from build123d import *

# Parameters (mm, degrees)
BOSS_EXTRUDE1_DEPTH   = 2.4
FILLET1_R             = 1
SKETCH3_R             = 1.9225
BOSS_EXTRUDE2_DEPTH   = 141
KES_EKSTR_ZYON1_DEPTH = 0.06


with BuildPart() as part:
    # Sketch1 → Boss-Extrude1 (new body)
    with BuildSketch(Plane(origin=(0, 0, 0), x_dir=(1, 0, 0), z_dir=(0, 1, 0))):
        with BuildLine():
            Line((-15, 3.25), (-9.45714016, 3.25))
            ThreePointArc((-9.45714016, 3.25), (-7.071067812, 7.071067812), (-3.25, 9.45714016))
            Line((-3.25, 9.45714016), (-3.25, 15))
            ThreePointArc((-3.25, 15), (0, 18.25), (3.25, 15))
            Line((3.25, 15), (3.25, 9.45714016))
            ThreePointArc((3.25, 9.45714016), (7.071067812, 7.071067812), (9.45714016, 3.25))
            Line((9.45714016, 3.25), (15, 3.25))
            ThreePointArc((15, 3.25), (18.25, 0), (15, -3.25))
            Line((15, -3.25), (9.45714016, -3.25))
            ThreePointArc((9.45714016, -3.25), (7.071067812, -7.071067812), (3.25, -9.45714016))
            Line((3.25, -9.45714016), (3.25, -15))
            ThreePointArc((3.25, -15), (0, -18.25), (-3.25, -15))
            Line((-3.25, -15), (-3.25, -9.45714016))
            ThreePointArc((-3.25, -9.45714016), (-7.071067812, -7.071067812), (-9.45714016, -3.25))
            Line((-9.45714016, -3.25), (-15, -3.25))
            ThreePointArc((-15, -3.25), (-18.25, 0), (-15, 3.25))
        make_face()
        with BuildLine():
            Line((-15, 1.42), (-9.5, 1.42))
            ThreePointArc((-9.5, 1.42), (-8.08, 0), (-9.5, -1.42))
            Line((-9.5, -1.42), (-15, -1.42))
            ThreePointArc((-15, -1.42), (-16.42, 0), (-15, 1.42))
        make_face(mode=Mode.SUBTRACT)
        with BuildLine():
            Line((1.42, 15), (1.42, 9.5))
            ThreePointArc((1.42, 9.5), (0, 8.08), (-1.42, 9.5))
            Line((-1.42, 9.5), (-1.42, 15))
            ThreePointArc((-1.42, 15), (0, 16.42), (1.42, 15))
        make_face(mode=Mode.SUBTRACT)
        with BuildLine():
            Line((15, -1.42), (9.5, -1.42))
            ThreePointArc((9.5, -1.42), (8.08, 0), (9.5, 1.42))
            Line((9.5, 1.42), (15, 1.42))
            ThreePointArc((15, 1.42), (16.42, 0), (15, -1.42))
        make_face(mode=Mode.SUBTRACT)
        with BuildLine():
            Line((-1.42, -15), (-1.42, -9.5))
            ThreePointArc((-1.42, -9.5), (0, -8.08), (1.42, -9.5))
            Line((1.42, -9.5), (1.42, -15))
            ThreePointArc((1.42, -15), (0, -16.42), (-1.42, -15))
        make_face(mode=Mode.SUBTRACT)
    extrude(amount=BOSS_EXTRUDE1_DEPTH)

    # Fillet1
    fillet1_edges = [part.edges().sort_by_distance(p)[0] for p in [
        (-9.45714016, 1.2, -3.25),
        (-3.25, 1.2, -9.45714016),
        (3.25, 1.2, -9.45714016),
        (9.45714016, 1.2, -3.25),
        (9.45714016, 1.2, 3.25),
        (3.25, 1.2, 9.45714016),
        (-3.25, 1.2, 9.45714016),
        (-9.45714016, 1.2, 3.25),
    ]]
    fillet(fillet1_edges, radius=FILLET1_R)

    # Sketch2 → Revolve1 (revolve)
    with BuildSketch(Plane.XY):
        with BuildLine():
            Line((1.925, 29.7), (2.464294328, 29.7))
            ThreePointArc((2.464294328, 29.7), (4.04285617, 29.138592921), (4.912445377, 27.70651401))
            Line((4.912445377, 27.70651401), (7.5, 15.2))
            Line((7.5, 15.2), (7.5, 2.4))
            Line((7.5, 2.4), (5.625, 2.4))
            Line((5.625, 2.4), (5.625, 15.2))
            Line((5.625, 15.2), (3.404891948, 26.194820827))
            ThreePointArc((3.404891948, 26.194820827), (2.889371485, 27.2829386), (1.925, 28.003874988))
            Line((1.925, 28.003874988), (1.925, 29.7))
        make_face()
    revolve(axis=Axis((0, 2.4, 0), (0, 1, 0)))

    # Sketch3 → Boss-Extrude2 (add)
    with BuildSketch(Plane(origin=(0, 2.4, 0), x_dir=(1, 0, 0), z_dir=(0, 1, 0))):
        Circle(SKETCH3_R)
    extrude(amount=BOSS_EXTRUDE2_DEPTH)

    # Sketch4 → Revolve2 (revolve)
    with BuildSketch(Plane(origin=(0, 0, 0), x_dir=(0, 0, -1), z_dir=(1, 0, 0))):
        with BuildLine():
            Line((6.922649731, 142.4), (3.230934575, 136.005761782))
            ThreePointArc((3.230934575, 136.005761782), (2.938114252, 135.712941459), (2.538114252, 135.605761782))
            Line((2.538114252, 135.605761782), (1.9225, 135.605761782))
            Line((1.9225, 135.605761782), (1.9225, 143.4))
            Line((1.9225, 143.4), (0, 143.4))
            Line((0, 143.4), (0, 144.9))
            Line((0, 144.9), (17.5, 144.9))
            Line((17.5, 144.9), (17.5, 143.4))
            Line((17.5, 143.4), (8.654700538, 143.4))
            ThreePointArc((8.654700538, 143.4), (7.654700538, 143.132050808), (6.922649731, 142.4))
        make_face()
    revolve(axis=Axis((0, 143.4, 0), (0, -1, 0)))

    # Çizim1 → Kes-Ekstrüzyon1 (cut)
    with BuildSketch(Plane.XZ.offset(-143.4)):
        Polygon((2.473531895, 11.056579199), (2.409957676, 10.172692481), (0.082320957, 10.339489356), (0.334567051, 13.859997168), (2.66220377, 13.693200293), (2.599313145, 12.809997168), (1.511715488, 12.887926856), (1.480270176, 12.451794043), (2.237008457, 12.397790137), (2.173434238, 11.513903418), (1.416695957, 11.567907324), (1.385934238, 11.134508887), align=None)
        Polygon((3.792276096, 9.57689352), (2.680752659, 10.121717739), (5.101358127, 12.856776332), (6.685244846, 12.080213832), (6.008487034, 8.490663051), (4.89764719, 9.034803676), (5.015225315, 9.640467739), (4.199014377, 10.040370082), align=None)
        Polygon((4.76639719, 10.68704977), (5.177920627, 10.485389614), (5.35702219, 11.371327114), align=None, mode=Mode.SUBTRACT)
        with BuildLine():
            Line((10.49023887, 8.045909213), (9.301469339, 7.814170932))
            add(Edge.make_bspline(
                [(9.301469339, 7.814170932), (9.295162601, 7.849093276), (9.282863589, 7.91719668), (9.259765757, 8.016165899), (9.231766875, 8.109044475), (9.199649304, 8.196046435), (9.163730366, 8.277260103), (9.122086055, 8.351638268), (9.078384744, 8.421598141), (9.044202502, 8.463454613), (9.027348245, 8.484092807)],
                knots=[0, 0, 0, 0, 0.000106452, 0.000207596, 0.000304698, 0.000397269, 0.000485696, 0.00057075, 0.000652855, 0.000732716, 0.000732716, 0.000732716, 0.000732716], degree=3))
            add(Edge.make_bspline(
                [(9.027348245, 8.484092807), (9.01594409, 8.496831925), (8.993668142, 8.52171548), (8.957180327, 8.554902215), (8.918891069, 8.58263641), (8.879448715, 8.606805989), (8.837738681, 8.624547904), (8.795060394, 8.639748228), (8.750352942, 8.648261409), (8.689312805, 8.653650441), (8.61134576, 8.649600922), (8.51970475, 8.622824869), (8.429383641, 8.578500593), (8.375376925, 8.535791651), (8.347172464, 8.513487338)],
                knots=[0, 0, 0, 0, 5.1274e-05, 0.000100155, 0.000147599, 0.000192969, 0.000238571, 0.000283319, 0.000328632, 0.000374616, 0.000467063, 0.000560776, 0.000659216, 0.00076682, 0.00076682, 0.00076682, 0.00076682], degree=3))
            add(Edge.make_bspline(
                [(8.347172464, 8.513487338), (8.32238698, 8.49082732), (8.275523945, 8.447982998), (8.221828166, 8.374475546), (8.186518469, 8.299074978), (8.171541706, 8.220584969), (8.176882746, 8.140146557), (8.201970979, 8.058369087), (8.24745169, 7.976028431), (8.288027536, 7.924336237), (8.309574808, 7.896885776)],
                knots=[0, 0, 0, 0, 0.000100546, 0.000190108, 0.000271179, 0.000348404, 0.000427163, 0.000510645, 0.000603011, 0.000707603, 0.000707603, 0.000707603, 0.000707603], degree=3))
            Line((8.309574808, 7.896885776), (8.728617776, 8.253038119))
            Line((8.728617776, 8.253038119), (9.527055276, 7.314463901))
            Line((9.527055276, 7.314463901), (8.085356058, 6.088096713))
            add(Edge.make_bspline(
                [(8.085356058, 6.088096713), (8.043412666, 6.130918963), (7.963019255, 6.212996893), (7.848036495, 6.330909372), (7.745125301, 6.439426088), (7.651824198, 6.535975119), (7.570495488, 6.623033205), (7.499975002, 6.699500807), (7.440576701, 6.765659164), (7.404913451, 6.806519435), (7.388774026, 6.825010776)],
                knots=[0, 0, 0, 0, 0.000179825, 0.000344674, 0.000494074, 0.000628484, 0.000747456, 0.000851473, 0.000940545, 0.001014176, 0.001014176, 0.001014176, 0.001014176], degree=3))
            add(Edge.make_bspline(
                [(7.388774026, 6.825010776), (7.362058603, 6.85691328), (7.309444418, 6.919743064), (7.236989178, 7.015916122), (7.169853497, 7.110629262), (7.110069184, 7.204873936), (7.055748887, 7.297651818), (7.008392801, 7.389665379), (6.967289467, 7.480685486), (6.932054654, 7.570889978), (6.904285219, 7.660554079), (6.881879716, 7.748984602), (6.867047818, 7.836567991), (6.8580281, 7.923104859), (6.855033423, 8.008796842), (6.859351934, 8.093567562), (6.869528685, 8.177437845), (6.89179563, 8.287308778), (6.930587621, 8.421570582), (6.989518301, 8.577515834), (7.059974362, 8.728287923), (7.144056677, 8.87248116), (7.238974286, 9.012055008), (7.347673596, 9.144627972), (7.468154157, 9.271895089), (7.556552427, 9.35016865), (7.601371683, 9.389854526)],
                knots=[0, 0, 0, 0, 0.000124813, 0.000245811, 0.00036112, 0.000473004, 0.00058052, 0.000683552, 0.000783294, 0.000880029, 0.000973863, 0.001064719, 0.001153502, 0.001240092, 0.001325585, 0.00141045, 0.001494477, 0.001578803, 0.001746506, 0.001913085, 0.002078523, 0.002245136, 0.00241332, 0.002584355, 0.002758907, 0.002938427, 0.002938427, 0.002938427, 0.002938427], degree=3))
            add(Edge.make_bspline(
                [(7.601371683, 9.389854526), (7.633267182, 9.416124727), (7.696616127, 9.468301038), (7.794804449, 9.540632275), (7.89522225, 9.606383047), (7.996644151, 9.666761034), (8.100532816, 9.720065252), (8.205586837, 9.768027651), (8.312583613, 9.809888085), (8.420955565, 9.84541849), (8.529824651, 9.873991879), (8.63797322, 9.895680951), (8.744963509, 9.908130177), (8.850675885, 9.915266481), (8.955311133, 9.911662891), (9.058901226, 9.902751782), (9.161192476, 9.884483788), (9.262208706, 9.859340021), (9.361575353, 9.826665303), (9.457961526, 9.785512166), (9.551318063, 9.73663609), (9.641991537, 9.680468107), (9.72947251, 9.615894492), (9.814300197, 9.543841789), (9.89671096, 9.464752006), (9.947642677, 9.406869871), (9.973441995, 9.377549838)],
                knots=[0, 0, 0, 0, 0.000123949, 0.000246181, 0.000365628, 0.000483921, 0.000600102, 0.000715741, 0.000830244, 0.0009446, 0.001057681, 0.001167748, 0.001275177, 0.00138063, 0.001485255, 0.001588921, 0.001692315, 0.001796601, 0.001901012, 0.002005762, 0.002110638, 0.002216866, 0.002325426, 0.002436499, 0.002550592, 0.002667712, 0.002667712, 0.002667712, 0.002667712], degree=3))
            add(Edge.make_bspline(
                [(9.973441995, 9.377549838), (10.008964061, 9.333535211), (10.080876677, 9.244429836), (10.173686342, 9.096785456), (10.258402353, 8.938194374), (10.331918381, 8.768701017), (10.393760496, 8.59235643), (10.441989787, 8.412398366), (10.475629511, 8.230183983), (10.485369339, 8.107330913), (10.49023887, 8.045909213)],
                knots=[0, 0, 0, 0, 0.000169553, 0.000343252, 0.000522153, 0.000708588, 0.000896894, 0.001082278, 0.001267051, 0.001451795, 0.001451795, 0.001451795, 0.001451795], degree=3))
        make_face()
    extrude(amount=-KES_EKSTR_ZYON1_DEPTH, mode=Mode.SUBTRACT)


solid = part.part
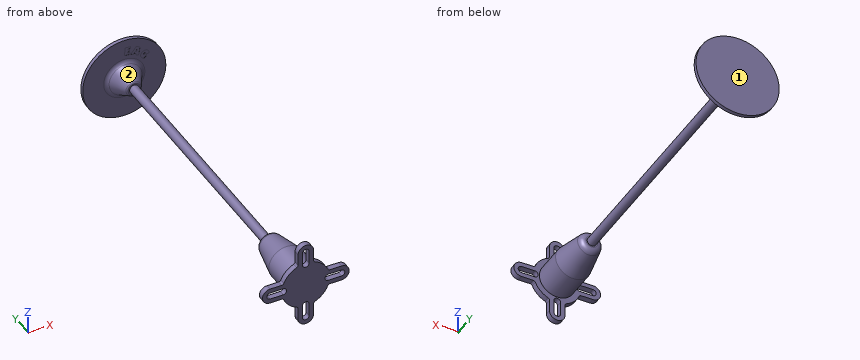
CAD build for the part. Positions are in the model's coordinates, mm. Face numbers are marked on the shaded views. A direction names the side the tool comes from. Round coordinates to 2 decimals unless told otherwise and drop trailing zeros. Order: outer loops, then holes, each group sorted by start corner. A loop starts at its lowest first (then second) coordinate and runs counter-clockwise, first axis right, second up. Notation, with made-up numbers: (2, -31.75) -> (29, -31.75) arc R23 ccw to (29, 7.25) -> close; hole circle Ø8 at (39, 67.5). An arc over 180 degrees is marked (long way). Write item = value, one per line. Start each with the question number.
(1) Cut at B-B, the plane x = -12.5. List the corners of the cut face in (y, z), then the cut area to 3 significant figures.
(2) Cut at D-D, the plane y = 51.5. List the corners of the cut face in (x, z) (1 decimal), then the cut area to 3 significant figures.
(3) Cut at A-A, the plane y = 11.5. State how many separate pieces and enclosed holes the cut face has, then the cut area to 3 significant figures.
(4) Which spindle directions (+Z, -Z, +X, -X, +Y, -Y) get a long thin tool onto all of the face, cutting with end or side? Do the marked faces 1 and 2. Say none if no direction does.
(5) Pin check, flat tips, straight feed: P1, Ø1.9, axis at y = 1, z = 12, coming from the +X side; P2, Ø2.5, axis at y = 1.5, z = -13, coming from the -X side; P3, Ø1.9, axis at x = 12.5, y = 1.5, coming from the +Z side. Stop position of each tip, or through.
(6) Probe line 1 (X direction, y = 8, z = 0) (1 decimal); line 2 (Y direction, x = 1.5, z = 1.5); line 3 (Y direction, x = -0.5, z = -16.5). List the from-to ranges inside material, lowest first. Write a range as [from, to].
Model answer:
q1.outline = (0, -3.25) -> (2.4, -3.25) -> (2.4, -1.42) -> (0, -1.42) -> close; (0, 1.42) -> (2.4, 1.42) -> (2.4, 3.25) -> (0, 3.25) -> close; (143.4, -12.25) -> (144.9, -12.25) -> (144.9, 12.25) -> (143.4, 12.25) -> close
q1.area = 45.5 mm2
q2.outline = circle Ø3.8 at (0, 0)
q2.area = 11.6 mm2
q3.separate_pieces = 2
q3.enclosed_holes = 1
q3.area = 88.9 mm2
q4.face_1 = +Z, -Z, +X, -X, +Y
q4.face_2 = none
q5.P1 = 3.25
q5.P2 = -3.25
q5.P3 = 3.25
q6.line_1 = [-7.5, -5.6], [-1.9, 1.9], [5.6, 7.5]
q6.line_2 = [0, 2.4], [27.91, 29.7], [135.61, 144.9]
q6.line_3 = [0, 2.4], [143.4, 144.9]
